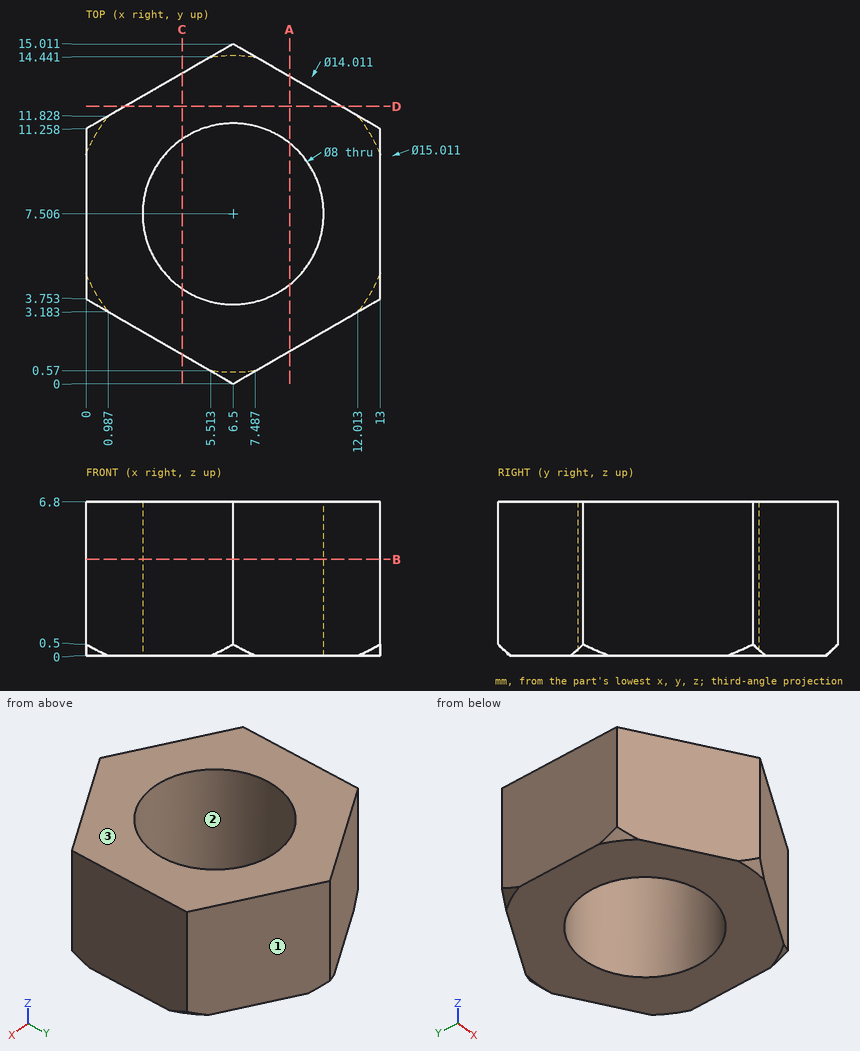
Geometry check sheet. Reference: drawing and pictorial views, mm from the part's lowest x, y, z. Give positions to 0.01 mm unless a question says otherwise; leave off trailing zeros. Write each loop counter-clockwise with the first axis right and the second up, starting at its lowest first coordinate (ties: lowest second). Pieces come first, ordered by that corner, then holes. Notation, with made-up numbers: M 78.5,35.5 L 118.5,35.5 A28 ccw 118.5,58.5 Z; hole C -27.75,9 d6. An arc over 180 degrees is marked long. Answer as CSV lines item,"result". Start each with the question number.
Q1. Go/stop test with flat-tipped pins: pin 1 (1.5 mm diameter, centred on x = 2, z = 6, fed in from +Y) (1 decimal); pin 2 (5 mm diameter, centred on x = 6.5, y = 7.51, fed in from +Z) (3 decimals). Record where each tip stops, or that it passes through.
Q2. Section check B-B, the plane z = 4.25. Record the cut outline in (x, y) (1 decimal).
Q3. Section check A-A, the plane x = 9. Record the cut outline in (y, z).
Q4. Section check C-C, the plane x = 4.25. Record the cut outline in (y, z).
Q5. Section check D-D, the plane y = 12.25. Record the cut outline in (x, z).
Q6. Material ranges on L1, parallel to X at y = 12.5, z = 0.75; L2, parallel to X at y = 13, z = 6.5 (1 decimal); L3, parallel to X at y = 4.75, z = 6.5, recorded low to high.
Q7. Release check for a two-part mould opening along X. For the marked faces 1, 2 and 3 record: pulls with the +X half, pulls with the -X half, needs draft (parallel to the pull), parting line crosses it, or undercut.
Geometry says:
1,pin 1,"y = 12.8"
1,pin 2,"through"
2,outline,"M 0,3.8 L 6.5,0 L 13,3.8 L 13,11.3 L 6.5,15 L 0,11.3 Z; hole C 6.5,7.5 d8"
3,outline,"M 1.44,0 L 4.38,0 L 4.38,6.8 L 1.44,6.8 Z; M 10.63,0 L 13.57,0 L 13.57,6.8 L 10.63,6.8 Z"
4,outline,"M 1.3,0 L 4.2,0 L 4.2,6.8 L 1.3,6.8 Z; M 10.81,0 L 13.71,0 L 13.71,6.8 L 10.81,6.8 Z"
5,outline,"M 1.72,0 L 11.28,0 L 11.28,6.8 L 1.72,6.8 Z"
6,L1,"2.15 to 10.85"
6,L2,"3 to 10"
6,L3,"0 to 3.6, 9.4 to 13"
7,face 1,"pulls with the +X half"
7,face 2,"undercut"
7,face 3,"needs draft"
